Part model, mm, in its own coordinate system. Give positions to 0.01 mm unless a question says otherwise; leave off trailing zeros. Order: outer loops, then holes, each group sorted by start corner. A loop starts at its lowest first (then second) coordinate and runs counter-clockwise, first axis right, second up.
from build123d import *

# Parameters (mm, degrees)
SKETCH1_W           = 262.6868
SKETCH1_H           = 130.175
BOSS_EXTRUDE1_DEPTH = 4.3434
SKETCH2_W           = 19.05
SKETCH2_H           = 8.6868
CUT_EXTRUDE1_DEPTH  = 147.650388692
CUT_EXTRUDE2_DEPTH  = 147.650388692
SKETCH3_W           = 8.6868
SKETCH3_H           = 19.05
CUT_EXTRUDE3_DEPTH  = 147.650388692
FILLET1_R           = 2.54


with BuildPart() as part:
    # Sketch1 → Boss-Extrude1 (new body)
    with BuildSketch(Plane.XY):
        Rectangle(SKETCH1_W, SKETCH1_H)
    extrude(amount=BOSS_EXTRUDE1_DEPTH)

    # Sketch2 → Cut-Extrude1 (cut, through all)
    with BuildSketch(Plane.XY.offset(4.3434)):
        with Locations((-50.8, 65.0875)):
            Rectangle(SKETCH2_W, SKETCH2_H)
        with Locations((0, 65.0875)):
            Rectangle(SKETCH2_W, SKETCH2_H)
        with Locations((50.8, 65.0875)):
            Rectangle(SKETCH2_W, SKETCH2_H)
        with Locations((101.6, 65.0875)):
            Rectangle(SKETCH2_W, SKETCH2_H)
        with Locations((-101.6, 65.0875)):
            Rectangle(SKETCH2_W, SKETCH2_H)
    extrude(amount=-CUT_EXTRUDE1_DEPTH, mode=Mode.SUBTRACT)

    # Sketch4 → Cut-Extrude2 (cut, through all)
    with BuildSketch(Plane.XY.offset(4.3434)):
        with BuildLine():
            Line((-19.05, -65.0875), (-19.05, -7.9375))
            ThreePointArc((-19.05, -7.9375), (0, 11.1125), (19.05, -7.9375))
            Line((19.05, -7.9375), (19.05, -65.0875))
            ThreePointArc((19.05, -65.0875), (0, -84.1375), (-19.05, -65.0875))
        make_face()
    extrude(amount=-CUT_EXTRUDE2_DEPTH, mode=Mode.SUBTRACT)

    # Sketch3 → Cut-Extrude3 (cut, through all)
    with BuildSketch(Plane.XY.offset(4.3434)):
        with Locations((-131.3434, -25.4)):
            Rectangle(SKETCH3_W, SKETCH3_H)
        with Locations((-131.3434, 25.4)):
            Rectangle(SKETCH3_W, SKETCH3_H)
    cut_extrude3 = extrude(amount=-CUT_EXTRUDE3_DEPTH, mode=Mode.SUBTRACT)

    # Mirror1: Cut-Extrude3 across plane
    add(cut_extrude3.mirror(Plane(origin=(0, 0, 0), x_dir=(0, 0, 1), z_dir=(1, 0, 0))), mode=Mode.SUBTRACT)

    # Fillet1
    fillet1_edges = [part.edges().sort_by_distance(p)[0] for p in [
        (19.05, -65.0875, 2.1717),
        (-19.05, -65.0875, 2.1717),
    ]]
    fillet(fillet1_edges, radius=FILLET1_R)


solid = part.part
Item 1: Band-saw the part on B-B on x = 54.5. List the corners of the cut face in (y, z).
Item 2: Band-saw the part on A-A on y = -49. List the corners of the cut face in (x, z).
Item 3: Drill centre lines: probe 1 along X at (y, z) = (-45, 2.85); probe 2 along X at (y, z) = (-27, 4); probe 3 along Y at (x, z) = (-103.5, 0.8). Where is each one in solid material? Low to high.
Item 4: Drop flat-ended pins along their axis: P1, Ø1.3, axis at y = -27, z = 2, coming from the +X side; P2, Ø2, axis at x = 97.5, z = 2.5, coming from the +Y side. Give the stop position or say it passes through.
Item 5: Band-saw the part on C-C on x = 0. List the corners of the cut face in (y, z).
Working result:
1. outline: (-65.09, 0) - (60.74, 0) - (60.74, 4.34) - (-65.09, 4.34) - close
2. outline: (-131.34, 0) - (-19.05, 0) - (-19.05, 4.34) - (-131.34, 4.34) - close; (19.05, 0) - (131.34, 0) - (131.34, 4.34) - (19.05, 4.34) - close
3. probe 1: x = -131.34 to -19.05, 19.05 to 131.34
3. probe 2: x = -127 to -19.05, 19.05 to 127
3. probe 3: y = -65.09 to 60.74
4. P1: stops at x = 127
4. P2: stops at y = 60.74
5. outline: (11.11, 0) - (60.74, 0) - (60.74, 4.34) - (11.11, 4.34) - close
